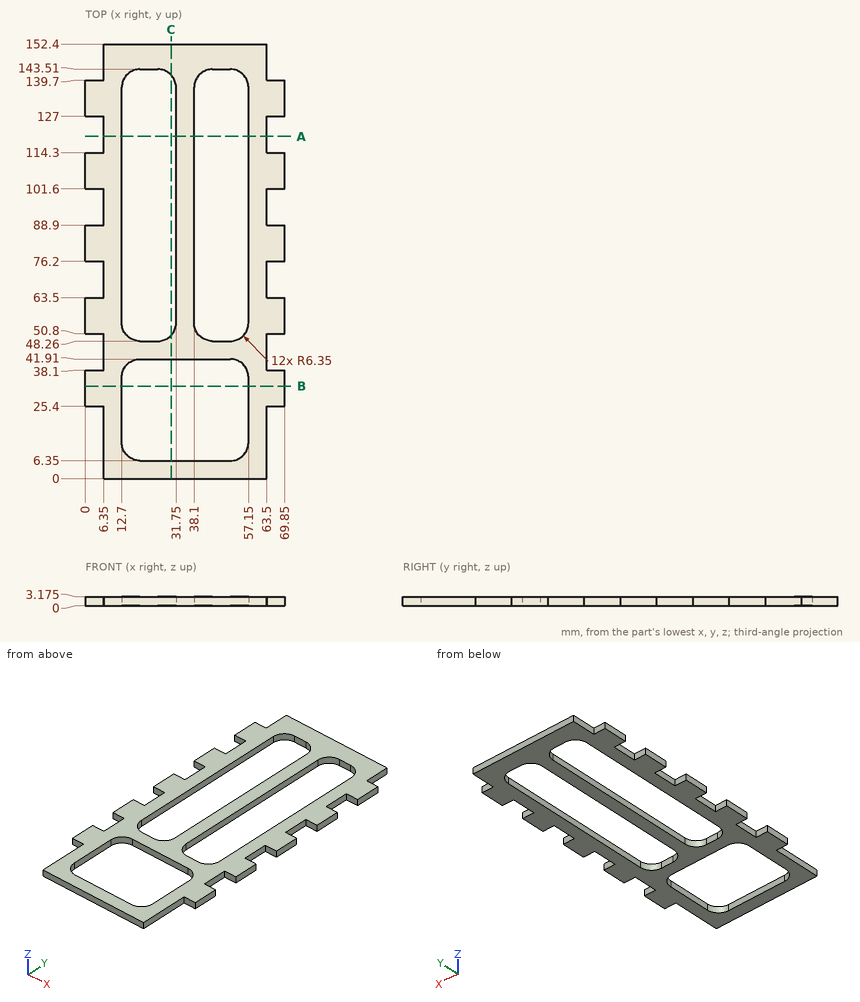
Geometry check sheet. Reference: drawing and pictorial views, mm from the part's lowest x, y, z. Give positions to 0.01 mm unless a question says otherwise; leave off trailing zeros. Order: outer loops, then holes, each group sorted by start corner. A loop starts at its lowest first (then second) coordinate and runs counter-clockwise, first axis right, second up. Notation, with made-up numbers: M 2,54.5 L 36,54.5 A4 ccw 36,59.5 Z; hole C -4,11.25 d7. An arc over 180 degrees is marked long. Answer in a Markdown table with one row per item.
1) Cross-section at C-C, the plane x = 30. Count the separate pieces of the cut face and the enclosed holes in it, plus the area to 3 significant figures.
Filled sheet:
| item | result |
|---|---|
| separate pieces | 3 |
| enclosed holes | 0 |
| area | 81.1 mm2 |
2) Thickness scan on L1, parallel to X at y = 81, z = 0.7; L2, parallel to X at y = 117, z = 1.7; L3, parallel to Y at x = 51, z = 2.9. Record the ranges inside material, lowest first. Write a range as [from, to].
Filled sheet:
| item | result |
|---|---|
| L1 | x = [0, 12.7], [31.75, 38.1], [57.15, 69.85] |
| L2 | x = [6.35, 12.7], [31.75, 38.1], [57.15, 63.5] |
| L3 | y = [0, 6.35], [41.91, 48.26], [143.51, 152.4] |
3) Cross-section at A-A, the plane y = 120. Enter the section's corners in (x, z) (3 decimals), plus the area to 3 significant figures.
Filled sheet:
| item | result |
|---|---|
| outline | M 6.35,0 L 12.7,0 L 12.7,3.175 L 6.35,3.175 Z; M 31.75,0 L 38.1,0 L 38.1,3.175 L 31.75,3.175 Z; M 57.15,0 L 63.5,0 L 63.5,3.175 L 57.15,3.175 Z |
| area | 60.5 mm2 |
4) Cross-section at B-B, the plane y = 32.5. Enter the section's corners in (x, z) (3 decimals).
Filled sheet:
| item | result |
|---|---|
| outline | M 0,0 L 12.7,0 L 12.7,3.175 L 0,3.175 Z; M 57.15,0 L 69.85,0 L 69.85,3.175 L 57.15,3.175 Z |
5) Gauge pin test, flat ends, axial feed: P1, Ø10, axis at x = 62, y = 53, coming from the -Z side; P2, Ø1, axis at y = 143.5, z = 1, coming from the -X side; P3, Ø1.6, axis at x = 65.5, z = 2, coming from the +Y side; P4, Ø1.6, axis at y = 71, z = 1, coming from the +X side. Record the tip position at first contact, or that the pin passes through.
Filled sheet:
| item | result |
|---|---|
| P1 | stops at z = 0 |
| P2 | stops at x = 6.35 |
| P3 | stops at y = 139.7 |
| P4 | stops at x = 63.5 |
